```python
from build123d import *

# Parameters (mm, degrees)
SKETCH1_W                 = 12.7
SKETCH1_H                 = 25.4
BOSS_EXTRUDE1_DEPTH       = 3.175
CHAMFER1_SIZE             = 3.175
F_2_CLEARANCE_SLOT1_DEPTH = 3.175


# Read off the part's stored shape, not the designer's step: #2 Clearance Slot1
with BuildPart() as part:
    # Sketch1 → Boss-Extrude1 (new body)
    with BuildSketch(Plane.XY):
        with Locations((119.14748118, -2406.283004154)):
            Rectangle(SKETCH1_W, SKETCH1_H)
    extrude(amount=BOSS_EXTRUDE1_DEPTH)

    # Chamfer1
    chamfer1_edges = [part.edges().sort_by_distance(p)[0] for p in [
        (125.49748118, -2393.583004154, 1.5875),
        (125.49748118, -2418.983004154, 1.5875),
    ]]
    chamfer(chamfer1_edges, length=CHAMFER1_SIZE)

    # #2 Clearance Slot1 outline → #2 Clearance Slot1 (cut)
    with BuildSketch(Plane.XY):
        with BuildLine():
            Line((117.32503118, -2414.455454154), (117.32503118, -2398.110554154))
            ThreePointArc((117.32503118, -2398.110554154), (115.97248118, -2396.758004154), (114.61993118, -2398.110554154))
            Line((114.61993118, -2398.110554154), (114.61993118, -2414.455454154))
            ThreePointArc((114.61993118, -2414.455454154), (115.97248118, -2415.808004154), (117.32503118, -2414.455454154))
        make_face()
    extrude(amount=F_2_CLEARANCE_SLOT1_DEPTH, mode=Mode.SUBTRACT)


solid = part.part
```
Can you work these out from the model? Positions are in its coordinate system, mm. A direction names the side the tool comes from. Give positions to 0.01 mm unless a question says otherwise; leave off trailing zeros. Write each loop counter-clockwise with the first axis right and the second up, starting at its lowest first coordinate (ties: lowest second). Pieces come first, ordered by that corner, then holes. Notation, with made-up numbers: (-30.5, -7) - (23.5, -7) arc R30 ccw to (23.5, 29) - close; hole circle Ø11 at (-9, 10). An arc over 180 degrees is marked (long way). Write item = value, one per line. Start each with the question number.
1. Thinking about a two-plate mould opening in Y: for faces 3 (the face through (119, -2406, 0)), 4 (the face through (123.89, -2395.15, 1.57)), 5 (the face through (117.325, -2406, 2)), 6 (the face through (115.943, -2415.808, 1.565)), which applies, released by +Y, released by -Y, zero draft, split by the parting line, or undercut?
2. Please list where these lines run through material, in increasing order: line 1 (X direction, y = -2406.25, z = 2.25); line 2 (X direction, y = -2415, z = 0.9); line 3 (Y direction, x = 115.25, z = 1.7).
3. Imagine slicing it at A-A (y = -2412). Please give me the cut outline in (x, z) (3 decimals), and give its area (3 significant figures).
4. Imagine slicing it at D-D (x = 123.75). Please give me the cut outline in (y, z) (3 decimals), and give its area (3 significant figures).
5. Imagine slicing it at C-C (x = 116.5). Please give me the cut outline in (y, z) (3 decimals), and give its area (3 significant figures).
6. On a 3-axis mill with a long thin cutter (end or side, diameter ignored), from which of +Z, -Z, +X, -X, +Y, -Y can I reach the whole of each face in a straight line? I mean faces 1 (the face through (116, -2396.76, 1.57)), 2 (the face through (117, -2393.583, 2)). Say none if no direction works.
7. Imagine slicing it at B-B (z = 2.3). Please give me the cut outline in (x, y), and give its area (3 significant figures).
Worked answers:
q1.face_3 = zero draft
q1.face_4 = released by +Y
q1.face_5 = undercut
q1.face_6 = undercut
q2.line_1 = 112.8 to 114.62, 117.33 to 125.5
q2.line_2 = 112.8 to 114.73, 117.21 to 125.5
q2.line_3 = -2418.98 to -2415.6, -2396.97 to -2393.58
q3.outline = (112.797, 0) - (114.62, 0) - (114.62, 3.175) - (112.797, 3.175) - close; (117.325, 0) - (125.497, 0) - (125.497, 3.175) - (117.325, 3.175) - close
q3.area = 31.7 mm2
q4.outline = (-2417.555, 0) - (-2395.011, 0) - (-2395.011, 3.175) - (-2417.555, 3.175) - close
q4.area = 71.6 mm2
q5.outline = (-2418.983, 0) - (-2415.701, 0) - (-2415.701, 3.175) - (-2418.983, 3.175) - close; (-2396.865, 0) - (-2393.583, 0) - (-2393.583, 3.175) - (-2396.865, 3.175) - close
q5.area = 20.8 mm2
q6.face_1 = +Z, -Z
q6.face_2 = +Z, -Z, +X, -X, +Y
q7.outline = (112.8, -2418.98) - (122.32, -2418.98) - (125.5, -2415.81) - (125.5, -2396.76) - (122.32, -2393.58) - (112.8, -2393.58) - close; hole (114.62, -2414.46) arc R1.35 ccw to (117.33, -2414.46) - (117.33, -2398.11) arc R1.35 ccw to (114.62, -2398.11) - close
q7.area = 263 mm2
